from build123d import *

# Parameters (mm, degrees)
F0_W     = 30
F0_H     = 25
F1_DEPTH = 2
F2_R     = 6
F3_DEPTH = 1.6


with BuildPart() as f1:
    # F0 (on Top) → F1 (new body)
    with BuildSketch(Plane.XY):
        Rectangle(F0_W, F0_H)
    extrude(amount=-F1_DEPTH)

    # F2 (on Top) → F3 (cut)
    with BuildSketch(Plane.XY):
        with Locations((-7.865239, -4.20318)):
            Circle(F2_R)
        with Locations((2.998843, 5.818724)):
            Circle(F2_R)
        with Locations((8.051903, -5.971751)):
            Circle(F2_R)
    extrude(amount=-F3_DEPTH, mode=Mode.SUBTRACT)


solid = f1.part
For this review, take the finished solid that the model builds, in its own axes (mm). A direction names the side the tool comes from. Round coordinates to 2 decimals unless told otherwise and drop trailing zeros. Loops run counter-clockwise (first coordinate to the right, second up) from the corner with the lowest first, then second, coordinate; pieces in that order, holes last. Notation, with made-up numbers: (19, 0) - (44, 0) arc R17 cw to (44, 5) - close; hole circle Ø4 at (-12, -39). An arc over 180 degrees is marked (long way). Use one line per item in the form item = value.
Item 1: Consider section C-C on y = -1. Write out the cut boundary in (x, z), then the cut area to 3 significant figures.
Answers:
outline = (-15, -2) - (15, -2) - (15, 0) - (11.41, 0) - (11.41, -1.6) - (4.69, -1.6) - (4.69, 0) - (-2.79, 0) - (-2.79, -1.6) - (-12.94, -1.6) - (-12.94, 0) - (-15, 0) - close
area = 33.0 mm^2
Item 2: Clearance check with a flat-ended pin moving along its axis: P1, Ø11, axis at x = 3, y = 5.82, coming from the +Z side. State where the tip first meets the part, or that it passes through.
Answers:
P1 = -1.6
Item 3: Tool access review of faces 4 (the flat face through (-8, -4, -1.6)), 5 (the flat face through (0, 12.5, -1)): name each direction out of +Z, -Z, +X, -X, +Y, -Y from which nothing blocks a thin tool from reaching the whole face with its end or side.
Answers:
face_4 = +Z
face_5 = +Z, -Z, +X, -X, +Y
Item 4: Consider section D-D on x = -9. Write out the cut boundary in (y, z), then the cut area to 3 significant figures.
Answers:
outline = (-12.5, -2) - (12.5, -2) - (12.5, 0) - (1.69, 0) - (1.69, -1.6) - (-10.09, -1.6) - (-10.09, 0) - (-12.5, 0) - close
area = 31.1 mm^2
Item 5: Mouldability with a two-part tool opening along X and no side actions: class faces 1 (the flat face through (-15, 0, -1)), 2 (the cylindrical face through (-13.86, -3.94, -0.79)), 3 (the flat face through (0, -12.5, -1)) as +X half, -X half, draft (parallel to the pull), parting line (faces both ways), or undercut.
Answers:
face_1 = -X half
face_2 = undercut
face_3 = draft
Item 6: Consider section B-B on x = -2.25. Write out the cut boundary in (y, z), then the cut area to 3 significant figures.
Answers:
outline = (-12.5, -2) - (12.5, -2) - (12.5, 0) - (8.73, 0) - (8.73, -1.6) - (2.91, -1.6) - (2.91, 0) - (-2.09, 0) - (-2.09, -1.6) - (-6.32, -1.6) - (-6.32, 0) - (-12.5, 0) - close
area = 33.9 mm^2
Item 7: For line 1 (X direction, y = 6, z = -0.65); line 2 (X direction, y = -4.75, z = -0.4); line 3 (X direction, y = -9, z = -0.3), list the stretches that pass through material, from the lowest coordinate up.
Answers:
line_1 = -15 to -3, 9 to 15
line_2 = -15 to -13.84, -1.89 to 2.18, 13.93 to 15
line_3 = -15 to -11.47, -4.26 to 2.87, 13.23 to 15
Item 8: Consider section A-A on z = -0.9. Write out the cut boundary in (x, y).
Answers:
outline = (-15, -12.5) - (15, -12.5) - (15, 12.5) - (-15, 12.5) - close; hole circle Ø12 at (-7.87, -4.2); hole circle Ø12 at (3, 5.82); hole circle Ø12 at (8.05, -5.97)
